For this review, take the finished solid that the model builds, in its own axes (mm). A direction names the side the tool comes from. Coordinates: 2 decimals unless noted, no trailing zeros. Order: outer loops, then holes, each group sorted by start corner. A loop starts at its lowest first (then second) coordinate and runs counter-clockwise, first axis right, second up. Notation, with made-up numbers: (17, 81.25) -> (74, 81.25) arc R21 ccw to (74, 106.25) -> close; hole circle Ø8 at (81.5, 89). An arc over 180 degrees is marked (long way). Answer as a JSON object with one key per item and string values. Group by question number.
1) Machinability: for faces 1 (the flat face through (-1, 1, -0.5)), 2 (the conical face through (26.416, -0.542, -0.707)), which of the approach directions +Z, -Z, +X, -X, +Y, -Y give a long, thin tool a straight path to every point of the face, cutting with its end or side? Answer none if there is none.
2) Add section A-A, the plane x = 19.25. Write out the cut boundary in (y, z), then the cut area to 3 significant figures.
3) Draft analysis for pull direction X (two halves, no side actions). For faces 3 (the flat face through (-0.6, 1.5, 0)), 4 (the cylindrical face through (3, -2, 0)), 5 (the flat face through (-1, -1, -0.5)), state which applies: +X half, -X half, draft (parallel to the pull), parting line (faces both ways), or undercut.
4) Wall thickness on L1, parallel to X at y = 3.75, z = -3; L2, parallel to Y at x = 15, z = 0; L3, parallel to X at y = -2.75, z = 0.5: over which ranges is each line inside the solid? List them lowest first.
5) Add section B-B, the plane z = 3.75. Write out the cut boundary in (x, y) (3 decimals), then the cut area to 3 significant figures.
6) For pin 1 (4 mm diameter, centred on x = 15, y = -3, fed in from +Z); pin 2 (1.6 mm diameter, centred on x = -1, z = -1.5, fed in from +Y); pin 3 (1.6 mm diameter, centred on x = -1, y = 2, fed in from +Z); pin 4 (2 mm diameter, centred on x = 5, z = -4, fed in from -Y), all flat-tipped, find the tip position at first contact; note any pin that passes through.
from build123d import *

# Parameters (mm, degrees)
F3_DEPTH = 0.5


# Not quite as in the source:
# - a pattern or mirror of a feature is missing from the dataset's text; its kind, count and spacing are read off the source's solid


with BuildPart() as f1:
    # F0 (on Front) → F1 (revolve)
    with BuildSketch(Plane.XZ):
        with BuildLine():
            Line((28, 0), (24, 2.25))
            Line((24, 2.25), (6, 2.25))
            Line((6, 2.25), (5.75, 2))
            Line((5.75, 2), (0.8660254038, 2))
            Line((0.8660254038, 2), (0, 2.5))
            Line((0, 2.5), (0, 5.5))
            Line((0, 5.5), (-1, 5.5))
            Line((-1, 5.5), (-1, 4.5))
            ThreePointArc((-1, 4.5), (-1.7469875145, 2.3048861143), (-2, 0))
            Line((-2, 0), (28, 0))
        make_face()
    revolve(axis=Axis((13, 0, 0), (-1, 0, 0)))

    # F2 (on Front) → F3 (cut, symmetric)
    with BuildSketch(Plane.XZ):
        Polygon((-1.7016947762, 2.5), (-2, 2.5), (-2, 0), (-2, -2.5), (-1.7016947762, -2.5), (0.5, -0.5), (0.5, 0), (0.5, 0.5), align=None)
    f3 = extrude(amount=F3_DEPTH, both=True, mode=Mode.SUBTRACT)

    # F3_copies: F3 across plane
    add(f3.mirror(Plane(origin=(0, 0, 0), x_dir=(0, -0.7071067802, -0.7071067821), z_dir=(-2.1e-09, -0.7071067821, 0.7071067802))), mode=Mode.SUBTRACT)


solid = f1.part
Output values:
{
 "1": {"face 1": "-X", "face 2": "+X"},
 "2": {"outline": "circle Ø4.5 at (0, 0)", "area": "15.9 mm²"},
 "3": {"face 3": "-X half", "face 4": "undercut", "face 5": "draft"},
 "4": {"L1": "x = -1 to 0", "L2": "y = -2.25 to 2.25", "L3": "x = -1.63 to 0"},
 "5": {"outline": "(-1, -4.023) -> (0, -4.023) -> (0, 4.023) -> (-1, 4.023) -> (-1, 2.487) arc R9.941 ccw to (-1, -2.487) -> close", "area": "9.10 mm²"},
 "6": {"pin 1": "stops at z = 2.02", "pin 2": "stops at y = 5.46", "pin 3": "stops at z = 5.37", "pin 4": "passes through"}
}
